from build123d import *

# Parameters (mm, degrees)
SKETCH_1_R      = 3
SKETCH_1_R_2    = 14.568467703
EXTRUDE_1_DEPTH = 5.75


with BuildPart() as part:
    # 草图1 → 凸台-拉伸1 (new body)
    with BuildSketch(Plane(origin=(0, 0, 0), x_dir=(1, 0, 0), z_dir=(0, 1, 0))):
        Polygon((0, 144.96), (0, 25.455844123), (25.455844123, 0), (144.96, 0), (144.96, 28.284271247), (28.284271247, 144.96), align=None)
        with Locations(Location((66.618795027, 15, 0), (0, 0, 270))):
            Circle(SKETCH_1_R, mode=Mode.SUBTRACT)
        with Locations(Location((15, 66.618795027, 0), (0, 0, 270))):
            Circle(SKETCH_1_R, mode=Mode.SUBTRACT)
        with Locations(Location((51.27, 51.27, 0), (0, 0, 270))):
            Circle(SKETCH_1_R_2, mode=Mode.SUBTRACT)
        with Locations(Location((101.618795027, 15, 0), (0, 0, 270))):
            Circle(SKETCH_1_R, mode=Mode.SUBTRACT)
        with BuildLine():
            ThreePointArc((90.868795027, 20), (86.618795027, 15.75), (82.368795027, 20))
            Line((82.368795027, 20), (82.368795027, 25))
            ThreePointArc((82.368795027, 25), (86.618795027, 29.25), (90.868795027, 25))
            Line((90.868795027, 25), (90.868795027, 20))
        make_face(mode=Mode.SUBTRACT)
        with BuildLine():
            ThreePointArc((120.868795027, 20), (116.618795027, 15.75), (112.368795027, 20))
            Line((112.368795027, 20), (112.368795027, 25))
            ThreePointArc((112.368795027, 25), (116.618795027, 29.25), (120.868795027, 25))
            Line((120.868795027, 25), (120.868795027, 20))
        make_face(mode=Mode.SUBTRACT)
        with BuildLine():
            Line((25, 82.368795027), (20, 82.368795027))
            ThreePointArc((20, 82.368795027), (15.75, 86.618795027), (20, 90.868795027))
            Line((20, 90.868795027), (25, 90.868795027))
            ThreePointArc((25, 90.868795027), (29.25, 86.618795027), (25, 82.368795027))
        make_face(mode=Mode.SUBTRACT)
        with Locations(Location((15, 101.618795027, 0), (0, 0, 270))):
            Circle(SKETCH_1_R, mode=Mode.SUBTRACT)
        with BuildLine():
            Line((25, 112.368795027), (20, 112.368795027))
            ThreePointArc((20, 112.368795027), (15.75, 116.618795027), (20, 120.868795027))
            Line((20, 120.868795027), (25, 120.868795027))
            ThreePointArc((25, 120.868795027), (29.25, 116.618795027), (25, 112.368795027))
        make_face(mode=Mode.SUBTRACT)
    extrude(amount=EXTRUDE_1_DEPTH)


solid = part.part
Model file for the job. Use its own axes, mm. A direction names the side the tool comes from. Round coordinates to 2 decimals unless told otherwise and drop trailing zeros. Order: outer loops, then holes, each group sorted by start corner. A loop starts at its lowest first (then second) coordinate and runs counter-clockwise, first axis right, second up. Notation, with made-up numbers: M 13.5,-21.75 L 66.5,-21.75 A19 ccw 66.5,-13.75 Z; hole C 82,42 d10. An arc over 180 degrees is marked long. Write each question's results on one line, items separated by ' | '. Start each with the question number.
(1) Saw through at C-C, the plane z = -51.27. Give the cut face in (x, y).
(2) Two-plate mould, pull along Z, no slides. Class faces 1 (the face through (84, 3, 0)), 2 (the face through (55, 5.75, -73)), 3 (the face through (22, 3, -90.869)): pulls with the +Z half, pulls with the -Z half, needs draft (parallel to the pull), parting line crosses it, or undercut.
(3) Saw through at A-A, the plane x = 55. Give the cut face in (y, z).
(4) Saw through at B-B, the plane y = 2.9. State how many separate pieces and enclosed holes the cut face has, then the cut area to 3 significant figures.
(5) Saw through at D-D, the plane z = -130. Give the cut face in (x, y), then the cut area to 3 significant figures.
(6) Drop flat-ended pins along their axis: pin 1 (1.5 mm diameter, centred on y = 4, z = -130.5, fed in from +X); pin 2 (1.5 mm diameter, centred on y = 2.5, z = -22, fed in from -X); pin 3 (2.5 mm diameter, centred on x = 22, y = 4, fed in from +Z); pin 4 (3.5 mm diameter, centred on x = 66.62, z = -15, fed in from -Y). Give the stop position or say it passes through.
(7) Probe probe 1 along X at (y, z) = (3.45, -15); probe 2 along Z at (x, y) = (20, 3.7); probe 3 along X at (y, z) = (1.4, -61.5). List the from-to ranges inside material, lowest first. Write a range as from..to.
(8) Which spindle directions (+Z, -Z, +X, -X, +Y, -Y) get a long thin tool onto all of the face, cutting with end or side? Do faces 4 (the face through (116.71, 2.83, -15.75)), 5 (the face through (87.439, 2.835, -85.805)). Say none if no direction does.
Established:
1) outline: M 0,0 L 36.7,0 L 36.7,5.75 L 0,5.75 Z; M 65.84,0 L 121.97,0 L 121.97,5.75 L 65.84,5.75 Z
2) face 1: pulls with the +Z half | face 2: needs draft | face 3: undercut
3) outline: M 0,-118.24 L 5.75,-118.24 L 5.75,-65.35 L 0,-65.35 Z; M 0,-37.19 L 5.75,-37.19 L 5.75,0 L 0,0 Z
4) separate pieces: 1 | enclosed holes: 9 | area: 12,700 mm^2
5) outline: M 0,0 L 43.24,0 L 43.24,5.75 L 0,5.75 Z | area: 249 mm^2
6) pin 1: stops at x = 43.49 | pin 2: stops at x = 2.71 | pin 3: stops at z = -2.21 | pin 4: passes through
7) probe 1: x = 10.46..63.62, 69.62..98.62, 104.62..144.96 | probe 2: z = -144.96..-120.87, -112.37..-90.87, -82.37..-5.46 | probe 3: x = 0..40.9, 61.64..111.74
8) face 4: +Y, -Y | face 5: -Z, +X, +Y, -Y
